```python
from build123d import *

# Parameters (mm, degrees)
SKETCH1_R           = 1.35
SKETCH1_R_2         = 1.353883359
BOSS_EXTRUDE1_DEPTH = 2.5
BOSS_EXTRUDE2_DEPTH = 1
CHAMFER1_SIZE       = 1
CHAMFER2_SIZE       = 2.5
CUT_EXTRUDE1_REACH  = 65.837


with BuildPart() as part:
    # Sketch1 → Boss-Extrude1 (new body)
    with BuildSketch(Plane.XY):
        with BuildLine():
            Line((-46.266968928, -27.305569911), (46.983031072, -27.305569911))
            ThreePointArc((46.983031072, -27.305569911), (52.736028884, -25.226770397), (55.831398017, -19.950684615))
            ThreePointArc((55.831398017, -19.950684615), (57.596036195, -0.805569911), (55.831398017, 18.339544793))
            ThreePointArc((55.831398017, 18.339544793), (52.736028884, 23.615630575), (46.983031072, 25.694430089))
            Line((46.983031072, 25.694430089), (-46.266968928, 25.694430089))
            ThreePointArc((-46.266968928, 25.694430089), (-52.019966741, 23.615630575), (-55.115335874, 18.339544793))
            ThreePointArc((-55.115335874, 18.339544793), (-56.879974052, -0.805569911), (-55.115335874, -19.950684615))
            ThreePointArc((-55.115335874, -19.950684615), (-52.019966741, -25.226770397), (-46.266968928, -27.305569911))
        make_face()
        with Locations((48.647296931, -19.366437107)):
            Circle(SKETCH1_R, mode=Mode.SUBTRACT)
        with Locations((48.647296931, 17.755297285)):
            Circle(SKETCH1_R, mode=Mode.SUBTRACT)
        with Locations((-47.931234788, 17.755297285)):
            Circle(SKETCH1_R, mode=Mode.SUBTRACT)
        with Locations((-47.931234788, -19.366437107)):
            Circle(SKETCH1_R_2, mode=Mode.SUBTRACT)
        with BuildLine():
            Line((-40.306968928, -14.970569911), (41.023031072, -14.970569911))
            ThreePointArc((41.023031072, -14.970569911), (44.558564977, -13.506103817), (46.023031072, -9.970569911))
            Line((46.023031072, -9.970569911), (46.023031072, 8.359430089))
            ThreePointArc((46.023031072, 8.359430089), (44.558564977, 11.894963995), (41.023031072, 13.359430089))
            Line((41.023031072, 13.359430089), (-40.306968928, 13.359430089))
            ThreePointArc((-40.306968928, 13.359430089), (-43.842502834, 11.894963995), (-45.306968928, 8.359430089))
            Line((-45.306968928, 8.359430089), (-45.306968928, -9.970569911))
            ThreePointArc((-45.306968928, -9.970569911), (-43.842502834, -13.506103817), (-40.306968928, -14.970569911))
        make_face(mode=Mode.SUBTRACT)
    extrude(amount=BOSS_EXTRUDE1_DEPTH)

    # Sketch2 → Boss-Extrude2 (add)
    with BuildSketch(Plane.XY.offset(2.5)):
        with BuildLine():
            Line((49.523031072, -9.970569911), (49.523031072, 8.359430089))
            ThreePointArc((49.523031072, 8.359430089), (47.033438712, 14.369837729), (41.023031072, 16.859430089))
            Line((41.023031072, 16.859430089), (-40.306968928, 16.859430089))
            ThreePointArc((-40.306968928, 16.859430089), (-46.317376569, 14.369837729), (-48.806968928, 8.359430089))
            Line((-48.806968928, 8.359430089), (-48.806968928, -9.970569911))
            ThreePointArc((-48.806968928, -9.970569911), (-46.317376569, -15.980977551), (-40.306968928, -18.470569911))
            Line((-40.306968928, -18.470569911), (41.023031072, -18.470569911))
            ThreePointArc((41.023031072, -18.470569911), (47.033438712, -15.980977551), (49.523031072, -9.970569911))
        make_face()
        with BuildLine():
            Line((41.023031072, 11.859430089), (-40.306968928, 11.859430089))
            ThreePointArc((-40.306968928, 11.859430089), (-42.781842663, 10.834303823), (-43.806968928, 8.359430089))
            Line((-43.806968928, 8.359430089), (-43.806968928, -9.970569911))
            ThreePointArc((-43.806968928, -9.970569911), (-42.781842663, -12.445443645), (-40.306968928, -13.470569911))
            Line((-40.306968928, -13.470569911), (41.023031072, -13.470569911))
            ThreePointArc((41.023031072, -13.470569911), (43.497904806, -12.445443645), (44.523031072, -9.970569911))
            Line((44.523031072, -9.970569911), (44.523031072, 8.359430089))
            ThreePointArc((44.523031072, 8.359430089), (43.497904806, 10.834303823), (41.023031072, 11.859430089))
        make_face(mode=Mode.SUBTRACT)
    extrude(amount=BOSS_EXTRUDE2_DEPTH)

    # Chamfer1
    chamfer1_edges = [part.edges().sort_by_distance(p)[0] for p in [
        (-42.781842663, 10.834303823, 3.5),
        (-43.806968928, -0.805569911, 3.5),
        (-42.781842663, -12.445443645, 3.5),
        (0.358031072, -13.470569911, 3.5),
        (43.497904806, -12.445443645, 3.5),
        (44.523031072, -0.805569911, 3.5),
        (43.497904806, 10.834303823, 3.5),
        (0.358031072, 11.859430089, 3.5),
        (49.523031072, -0.805569911, 3.5),
        (47.033438712, -15.980977551, 3.5),
        (0.358031072, -18.470569911, 3.5),
        (-46.317376569, -15.980977551, 3.5),
        (-48.806968928, -0.805569911, 3.5),
        (-46.317376569, 14.369837729, 3.5),
        (0.358031072, 16.859430089, 3.5),
        (47.033438712, 14.369837729, 3.5),
    ]]
    chamfer(chamfer1_edges, length=CHAMFER1_SIZE - 0.0001)  # a hair under: the kernel refuses the full size

    # Chamfer2
    chamfer2_edges = [part.edges().sort_by_distance(p)[0] for p in [
        (0.358031072, -27.305569911, 2.5),
        (52.736028884, -25.226770397, 2.5),
        (-52.019966741, -25.226770397, 2.5),
        (57.596036195, -0.805569911, 2.5),
        (-56.879974052, -0.805569911, 2.5),
        (52.736028884, 23.615630575, 2.5),
        (-52.019966741, 23.615630575, 2.5),
        (0.358031072, 25.694430089, 2.5),
    ]]
    chamfer(chamfer2_edges, length=CHAMFER2_SIZE - 0.0001)  # a hair under: the kernel refuses the full size

    # Sketch5 → Cut-Extrude1 (cut, up to next)
    with BuildSketch(Plane(origin=(0, 0, 0), x_dir=(1, 0, 0), z_dir=(0, 1, 0)), mode=Mode.PRIVATE) as cut_extrude1_sk1:
        with BuildLine():
            Line((-19.592815412, -0.909530151), (-10.792772138, -0.909530149))
            add(Edge.make_bspline(
                [(-10.792772138, -0.909530149), (-10.607889911, -0.909514148), (-10.425811047, -0.891482678), (-10.067163044, -0.820012158), (-9.888892808, -0.766003184), (-9.551032167, -0.625859061), (-9.390406566, -0.539750951), (-9.085426061, -0.336116729), (-8.94182552, -0.218381132), (-8.684308041, 0.03965313), (-8.5680613, 0.180457001), (-8.362346878, 0.487291556), (-8.276792708, 0.648789775), (-8.136603309, 0.98510143), (-8.08283068, 1.162298316), (-8.011186114, 1.523060599), (-7.992824871, 1.70562035), (-7.992815412, 1.890469849)],
                knots=[0, 0, 0, 0, 0.125, 0.125, 0.25, 0.25, 0.375, 0.375, 0.5, 0.5, 0.625, 0.625, 0.75, 0.75, 0.875, 0.875, 1, 1, 1, 1], degree=3))
            Line((-7.992815412, 1.890469849), (-7.992815414, 4.590513396))
            add(Edge.make_bspline(
                [(-7.992815414, 4.590513396), (-7.992831516, 4.77539614), (-8.010862926, 4.957475483), (-8.082333794, 5.316124243), (-8.136342538, 5.494395104), (-8.276486434, 5.832256678), (-8.36259727, 5.992880987), (-8.566235233, 6.297859231), (-8.683965434, 6.441464903), (-8.94199783, 6.698983866), (-9.082807296, 6.815224132), (-9.389639852, 7.020938991), (-9.551138299, 7.106493896), (-9.887450056, 7.246680754), (-10.064645109, 7.300455528), (-10.425407019, 7.372099354), (-10.607966433, 7.390460335), (-10.792815412, 7.39046985)],
                knots=[0, 0, 0, 0, 0.125, 0.125, 0.25, 0.25, 0.375, 0.375, 0.5, 0.5, 0.625, 0.625, 0.75, 0.75, 0.875, 0.875, 1, 1, 1, 1], degree=3))
            Line((-10.792815412, 7.39046985), (-19.592859134, 7.390469847))
            add(Edge.make_bspline(
                [(-19.592859134, 7.390469847), (-19.777741324, 7.39045368), (-19.95982018, 7.372422237), (-20.318468162, 7.300951771), (-20.496738382, 7.246942784), (-20.834598951, 7.106798619), (-20.995224508, 7.020690495), (-21.300204927, 6.817056293), (-21.443805472, 6.699320682), (-21.701322913, 6.441286422), (-21.817569624, 6.300482564), (-22.023283979, 5.993648079), (-22.108838169, 5.832149812), (-22.249027542, 5.495838191), (-22.302800153, 5.318641354), (-22.374444712, 4.957879073), (-22.392805954, 4.775319331), (-22.392815413, 4.590469849)],
                knots=[0, 0, 0, 0, 0.125, 0.125, 0.25, 0.25, 0.375, 0.375, 0.5, 0.5, 0.625, 0.625, 0.75, 0.75, 0.875, 0.875, 1, 1, 1, 1], degree=3))
            Line((-22.392815413, 4.590469849), (-22.39281541, 1.890426302))
            add(Edge.make_bspline(
                [(-22.39281541, 1.890426302), (-22.392799308, 1.705543556), (-22.374767902, 1.523464217), (-22.303297034, 1.164815473), (-22.249288291, 0.986544615), (-22.109144391, 0.648683022), (-22.023033556, 0.488058712), (-21.819395604, 0.183080482), (-21.701665392, 0.039474796), (-21.443632989, -0.218044171), (-21.302823525, -0.334284433), (-20.995990998, -0.539999282), (-20.834492517, -0.625554209), (-20.498180754, -0.765741045), (-20.320985718, -0.819515805), (-19.960223809, -0.89115971), (-19.777664402, -0.909520761), (-19.592815412, -0.909530151)],
                knots=[0, 0, 0, 0, 0.125, 0.125, 0.25, 0.25, 0.375, 0.375, 0.5, 0.5, 0.625, 0.625, 0.75, 0.75, 0.875, 0.875, 1, 1, 1, 1], degree=3))
        make_face()
    cut_extrude1_tool1 = extrude(cut_extrude1_sk1.sketch, amount=-CUT_EXTRUDE1_REACH, mode=Mode.PRIVATE) & part.part
    add(cut_extrude1_tool1.solids().sort_by_distance((-15.192815, 0, -3.240461))[0], mode=Mode.SUBTRACT)


solid = part.part
```
Can you work these out from the model? Positions are in its coordinate system, mm. A direction names the side the tool comes from. Give positions to 0.01 mm unless a question says otherwise; leave off trailing zeros. Order: outer loops, then holes, each group sorted by start corner. A loop starts at its lowest first (then second) coordinate and runs counter-clockwise, first axis right, second up. Notation, with made-up numbers: M 23.5,71.5 L 42.5,71.5 A7 ccw 42.5,84.5 Z; hole C 57.5,82.25 d6. An arc over 180 degrees is marked long. One line per item, written item: value.
1) We'd pull the mould along Y, two halves only. Please class faces 4 (the face through (44.597, 11.856, 1.232)), 5 (the face through (1.011, 24.462, 1.233)), 6 (the face through (-15, -21, 0.91)): released by +Y, released by -Y, zero draft, split by the parting line, or undercut.
Answer sheet:
face 4: undercut
face 5: released by +Y
face 6: zero draft
2) On a 3-axis mill with a long thin cutter (end or side, diameter ignored), from which of +Z, -Z, +X, -X, +Y, -Y can I reach the whole of each face in a straight line? I mean faces 1 (the face through (-46.68, -19.88, 1.23)), 2 (the face through (43.719, 10.996, 2.771)), 3 (the face through (-10, -14, 2.5)). Say none if no direction works.
Answer sheet:
face 1: +Z, -Z
face 2: +Z
face 3: -Z
3) Please list where these lines run through material, in increasing order: line 1 along X through (y, z) = (10, 1.8); line 2 along Y through (x, z) = (31.5, 0.55); line 3 along X through (y, z) = (10, 0.55).
Answer sheet:
line 1: x = -54.51 to -45.03, 45.75 to 55.23
line 2: y = -26.76 to -14.97, 13.36 to 25.14
line 3: x = -55.77 to -45.03, 45.75 to 56.48
4) For P1, Ø0.8, axis at x = 4, z = 1.5, coming from the -Y side; P2, Ø0.8, axis at y = -5, z = 1, coming from the +X side; P3, Ø2, axis at x = 30, y = 14, coming from the -Z side; P4, Ø1.5, axis at y = -21.5, z = 1.5, coming from the +X side, each with a flat end and sliding along its axis, tell me the tip position at first contact or that it passes through.
Answer sheet:
P1: stops at y = -26.21
P2: stops at x = 56.91
P3: stops at z = 0
P4: stops at x = 54.64
5) I want a section at B-B, the plane z = 1.85. List the corners of the cut face in (x, y) for me.
Answer sheet:
outline: M -53.3,-19.61 A7.15 ccw -46.27,-25.46 L 46.98,-25.46 A7.15 ccw 54.01,-19.61 A102.89 ccw 54.01,18 A7.15 ccw 46.98,23.84 L -46.27,23.84 A7.15 ccw -53.3,18 A102.89 ccw Z; hole C -47.93,-19.37 d2.71; hole C -47.93,17.76 d2.7; hole M -45.31,-9.97 A5 ccw -40.31,-14.97 L 41.02,-14.97 A5 ccw 46.02,-9.97 L 46.02,8.36 A5 ccw 41.02,13.36 L -40.31,13.36 A5 ccw -45.31,8.36 Z; hole C 48.65,-19.37 d2.7; hole C 48.65,17.76 d2.7
